Input: part model. Units: mm. Frame: model coordinates. Coordinates: 2 decimals unless noted, no trailing zeros. Order: outer loops, then holes, each group sorted by start corner. A loop starts at its lowest first (then second) coordinate and runs counter-clockwise, first axis right, second up. Notation, with made-up numbers: M 39,40.25 L 84,40.25 A25 ccw 84,72.25 Z; hole C 0,72.5 d8. An arc over 180 degrees is marked long. Answer in a Markdown table with one row per item.
from build123d import *

# Parameters (mm, degrees)
F1_W     = 50
F1_H     = 50
F4_W     = 50
F4_H     = 50
F5_DEPTH = 450


with BuildPart() as f2:
    # F2: sweep along a path in F0
    with BuildLine(Plane.XY) as f2_path:
        Line((-969.0792792215, 199.0843022242), (1030.9207207785, 199.0843022242))
        Line((1030.9207207785, 199.0843022242), (1030.9207207785, -400.9156977758))
        Line((1030.9207207785, -400.9156977758), (-969.0792792215, -400.9156977758))
        Line((-969.0792792215, -400.9156977758), (-969.0792792215, 199.0843022242))
    # F1 (on Right) → F2 (sweep)
    with BuildSketch(Plane.YZ):
        with Locations((199.0843022242, 0)):
            Rectangle(F1_W, F1_H)
    sweep(path=f2_path.line, transition=Transition.RIGHT)


with BuildPart() as f3_1:
    # F3: copy of F2
    add(f2.part.moved(Location((0, 0, 500))))


with BuildPart() as f2_1:
    add(f2.part)

    add(f3_1.part)  # F5 merges F3_1
    # F4 (on face) → F5 (join, through all)
    with BuildSketch(Plane.XY.offset(25)):
        with Locations((-969.0792792215, 199.0843022242)):
            Rectangle(F4_W, F4_H)
        with Locations((-969.0792792215, -400.9156977758)):
            Rectangle(F4_W, F4_H)
        with Locations((1030.9207207785, -400.9156977758)):
            Rectangle(F4_W, F4_H)
        with Locations((1030.9207207785, 199.0843022242)):
            Rectangle(F4_W, F4_H)
    extrude(amount=F5_DEPTH)


solid = f2_1.part
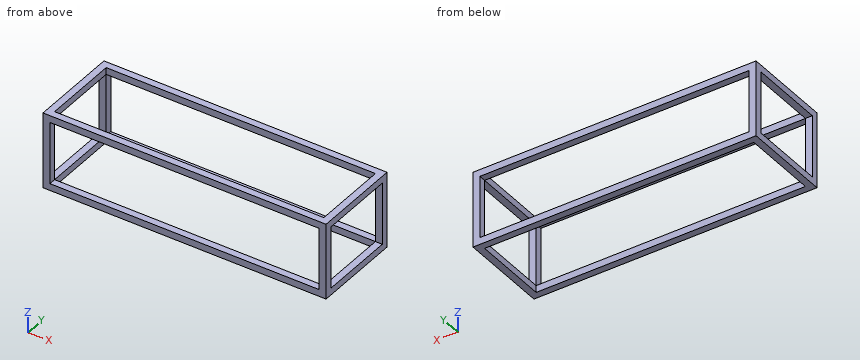
1) Cut plane A-A, the plane y = 107. Output: boundary loops of the cut face in (x, z), and give its area (3 significant figures).
Resolved:
| item | result |
|---|---|
| outline | M -994.08,-25 L -944.08,-25 L -944.08,25 L -994.08,25 Z; M -994.08,475 L -944.08,475 L -944.08,525 L -994.08,525 Z; M 1005.92,-25 L 1055.92,-25 L 1055.92,25 L 1005.92,25 Z; M 1005.92,475 L 1055.92,475 L 1055.92,525 L 1005.92,525 Z |
| area | 10,000 mm2 |
2) Material intervals for probe 1 along X at (y, z) = (186.5, 166); probe 2 along Z at (x, y) = (882.5, -391.5), sorted ascending.
Resolved:
| item | result |
|---|---|
| probe 1 | x = -994.08 to -944.08, 1005.92 to 1055.92 |
| probe 2 | z = -25 to 25, 475 to 525 |
3) Cut plane B-B, the plane x = -604. Output: boundary loops of the cut face in (y, z), and give its area (3 significant figures).
Resolved:
| item | result |
|---|---|
| outline | M -425.92,-25 L -375.92,-25 L -375.92,25 L -425.92,25 Z; M -425.92,475 L -375.92,475 L -375.92,525 L -425.92,525 Z; M 174.08,-25 L 224.08,-25 L 224.08,25 L 174.08,25 Z; M 174.08,475 L 224.08,475 L 224.08,525 L 174.08,525 Z |
| area | 10,000 mm2 |
